from build123d import *

# Parameters (mm, degrees)
SKETCH_1_W      = 50
SKETCH_1_H      = 50
SKETCH_1_R      = 1.65
EXTRUDE_2_DEPTH = 3
FILLET_1_R      = 2
FILLET_2_R      = 2
FILLET_3_R      = 2
FILLET_4_R      = 2


with BuildPart() as part:
    # 草图1 → 凸台-拉伸2 (new body)
    with BuildSketch(Plane(origin=(0, 0, 0), x_dir=(1, 0, 0), z_dir=(0, 1, 0))):
        Rectangle(SKETCH_1_W, SKETCH_1_H)
        with Locations((21.75, 21.75)):
            Circle(SKETCH_1_R, mode=Mode.SUBTRACT)
        with Locations((-21.75, 21.75)):
            Circle(SKETCH_1_R, mode=Mode.SUBTRACT)
        with Locations((21.75, -21.75)):
            Circle(SKETCH_1_R, mode=Mode.SUBTRACT)
        with Locations((-21.75, -21.75)):
            Circle(SKETCH_1_R, mode=Mode.SUBTRACT)
        with Locations((8, 0)):
            Circle(SKETCH_1_R, mode=Mode.SUBTRACT)
        with Locations((0, 8)):
            Circle(SKETCH_1_R, mode=Mode.SUBTRACT)
        with Locations((-8, 0)):
            Circle(SKETCH_1_R, mode=Mode.SUBTRACT)
        with Locations((0, -8)):
            Circle(SKETCH_1_R, mode=Mode.SUBTRACT)
    extrude(amount=EXTRUDE_2_DEPTH)

    # 圆角1
    fillet_1_edges = [part.edges().sort_by_distance(p)[0] for p in [
        (25, 1.5, 25),
    ]]
    fillet(fillet_1_edges, radius=FILLET_1_R)

    # 圆角2
    fillet_2_edges = [part.edges().sort_by_distance(p)[0] for p in [
        (25, 1.5, -25),
    ]]
    fillet(fillet_2_edges, radius=FILLET_2_R)

    # 圆角3
    fillet_3_edges = [part.edges().sort_by_distance(p)[0] for p in [
        (-25, 1.5, -25),
    ]]
    fillet(fillet_3_edges, radius=FILLET_3_R)

    # 圆角4
    fillet_4_edges = [part.edges().sort_by_distance(p)[0] for p in [
        (-25, 1.5, 25),
    ]]
    fillet(fillet_4_edges, radius=FILLET_4_R)


solid = part.part
The model under review builds one solid part; all positions refer to its coordinate system, in mm. Coordinates: 2 decimals unless noted, no trailing zeros. Write each loop counter-clockwise with the first axis right and the second up, starting at its lowest first coordinate (ties: lowest second). Pieces come first, ordered by that corner, then holes. Notation, with made-up numbers: (68.25, 80.25) - (82.25, 80.25) arc R26 ccw to (82.25, 112.25) - close; hole circle Ø9 at (-18.5, 88). An arc over 180 degrees is marked (long way). Answer as a JSON object with one key per item and string values. Group by question number.
1. Add section A-A (x = 0). Give the boundary of the cut face in (y, z).
2. Mouldability with a two-part tool opening along X and no side actions: class faces 1 (the face through (-24.4, 1.52, -24.43)), 2 (the face through (-9.65, 1.48, -0.07)), 3 (the face through (0, 1, -25)) as pulls with the +X half, pulls with the -X half, needs draft (parallel to the pull), parting line crosses it, or undercut.
3. Add section C-C (z = 8). Give the boundary of the cut face in (x, y), plus the area to 3 significant figures.
4. To check wall thickness, follow probe 1 along X at (y, z) = (1.75, 21.75); probe 2 along X at (y, z) = (1.65, 0); probe 3 along Z at (x, y) = (8, 1.3). State the ranges of each line that lie inside material, in increasing order.
5. Add section D-D (x = 7). Give the boundary of the cut face in (y, z), plus the area to 3 significant figures.
6. Clearance check with a flat-ended pin moving along its axis: pin 1 Ø2.5 at (x, z) = (-8, 0) entering from +Y. State where the tip first meets the part, or that it passes through.
7. Add section B-B (y = 2.5). Give the number of separate pieces and of enclosed holes in the cut face, plus the area to 3 significant figures.
Findings:
{
 "1": {"outline": "(0, -25) - (3, -25) - (3, -9.65) - (0, -9.65) - close; (0, -6.35) - (3, -6.35) - (3, 6.35) - (0, 6.35) - close; (0, 9.65) - (3, 9.65) - (3, 25) - (0, 25) - close"},
 "2": {"face 1": "pulls with the -X half", "face 2": "undercut", "face 3": "needs draft"},
 "3": {"outline": "(-25, 0) - (-1.65, 0) - (-1.65, 3) - (-25, 3) - close; (1.65, 0) - (25, 0) - (25, 3) - (1.65, 3) - close", "area": "140 mm²"},
 "4": {"probe 1": "-25 to -23.4, -20.1 to 20.1, 23.4 to 25", "probe 2": "-25 to -9.65, -6.35 to 6.35, 9.65 to 25", "probe 3": "-25 to -1.65, 1.65 to 25"},
 "5": {"outline": "(0, -25) - (3, -25) - (3, -1.31) - (0, -1.31) - close; (0, 1.31) - (3, 1.31) - (3, 25) - (0, 25) - close", "area": "142 mm²"},
 "6": {"pin 1": "through"},
 "7": {"separate pieces": "1", "enclosed holes": "8", "area": "2,430 mm²"}
}
